```python
from build123d import *

# Parameters (mm, degrees)
BOSS_EXTRUDE1_DEPTH = 11.1125
BOSS_EXTRUDE2_DEPTH = 12.7
CUT_EXTRUDE2_DEPTH  = 8
CUT_EXTRUDE3_DEPTH  = 96.942967533
SKETCH5_W           = 25.144717139
SKETCH5_H           = 15.875
CUT_EXTRUDE4_DEPTH  = 3.175
CUT_EXTRUDE5_DEPTH  = 96.942967533
SKETCH6_R           = 2.54
CUT_EXTRUDE6_DEPTH  = 96.942967533
CUT_EXTRUDE7_START  = -3.175
CUT_EXTRUDE7_DEPTH  = 3.175
CHAMFER1_SIZE       = 3.175
FILLET1_R           = 0.635
FILLET3_R           = 1.016
SKETCH8_R           = 2.286
CUT_EXTRUDE8_DEPTH  = 93.295392221


with BuildPart() as part:
    # Sketch3 → Boss-Extrude1 (new, symmetric)
    with BuildSketch(Plane(origin=(0, 0, 0), x_dir=(1, 0, 0), z_dir=(0, 1, 0))):
        Polygon((-56.934473853, -15.948934871), (-65.016704362, -7.866704362), (-82.294717139, -25.144717139), (-74.93090712, -32.508527158), (-74.21248663, -33.226947648), align=None)
        Polygon((-65.016704362, -7.866704362), (-55.873813681, -17.009595043), (-52.371513794, -13.507295156), (-61.514404475, -4.364404475), align=None)
        Polygon((-52.371513794, -13.507295156), (-51.564218639, -12.7), (-17.311249955, -12.7), (0, -12.7), (0, 0), (-17.311249955, 0), (-57.15, 0), (-60.325, -3.175), (-61.514404475, -4.364404475), align=None)
        Polygon((0, 0), (0, -12.7), (17.311249955, -12.7), (51.564218639, -12.7), (52.371513794, -13.507295156), (61.514404475, -4.364404475), (60.325, -3.175), (57.15, 0), (17.311249955, 0), align=None)
        Polygon((61.514404475, -4.364404475), (65.016704362, -7.866704362), (55.873813681, -17.009595043), (52.371513794, -13.507295156), align=None)
        Polygon((65.016704362, -7.866704362), (56.934473853, -15.948934871), (74.21248663, -33.226947648), (74.93090712, -32.508527158), (82.294717139, -25.144717139), align=None)
    extrude(amount=BOSS_EXTRUDE1_DEPTH, both=True)

    # Sketch2 → Boss-Extrude2 (add)
    with BuildSketch(Plane.XY):
        with BuildLine():
            Line((-50.804788276, 11.1125), (50.804788276, 11.1125))
            Line((50.804788276, 11.1125), (8.344749207, 34.318436746))
            ThreePointArc((8.344749207, 34.318436746), (0, 36.45), (-8.344749207, 34.318436746))
            Line((-8.344749207, 34.318436746), (-50.804788276, 11.1125))
        make_face()
    extrude(amount=BOSS_EXTRUDE2_DEPTH)

    # Sketch2<3> → Cut-Extrude2 (cut)
    with BuildSketch(Plane.XY):
        with BuildLine():
            ThreePointArc((0, 30.1), (-11.05, 19.05), (0, 8))
            Line((0, 8), (0, 10))
            ThreePointArc((0, 10), (-9.05, 19.05), (0, 28.1))
            Line((0, 28.1), (0, 30.1))
        make_face()
        with BuildLine():
            Line((0, 10), (0, 8))
            ThreePointArc((0, 8), (7.813529932, 11.236470068), (11.05, 19.05))
            ThreePointArc((11.05, 19.05), (7.813529932, 26.863529932), (0, 30.1))
            Line((0, 30.1), (0, 28.1))
            ThreePointArc((0, 28.1), (6.39931637, 25.44931637), (9.05, 19.05))
            ThreePointArc((9.05, 19.05), (6.39931637, 12.65068363), (0, 10))
        make_face()
        with BuildLine():
            ThreePointArc((0, 28.1), (-9.05, 19.05), (0, 10))
            Line((0, 10), (0, 28.1))
        make_face()
        with BuildLine():
            Line((0, 28.1), (0, 10))
            ThreePointArc((0, 10), (6.39931637, 12.65068363), (9.05, 19.05))
            ThreePointArc((9.05, 19.05), (6.39931637, 25.44931637), (0, 28.1))
        make_face()
    extrude(amount=CUT_EXTRUDE2_DEPTH, mode=Mode.SUBTRACT)

    # Sketch2<5> → Cut-Extrude3 (cut, through all)
    with BuildSketch(Plane.XY):
        with BuildLine():
            ThreePointArc((0, 28.1), (-9.05, 19.05), (0, 10))
            Line((0, 10), (0, 28.1))
        make_face()
        with BuildLine():
            Line((0, 28.1), (0, 10))
            ThreePointArc((0, 10), (6.39931637, 12.65068363), (9.05, 19.05))
            ThreePointArc((9.05, 19.05), (6.39931637, 25.44931637), (0, 28.1))
        make_face()
    extrude(amount=CUT_EXTRUDE3_DEPTH, mode=Mode.SUBTRACT)

    # Sketch5 → Cut-Extrude4 (cut)
    # profile 1 of 5: a face of its own
    with BuildSketch(Plane(origin=(0, 0, 0), x_dir=(-1, 0, 0), z_dir=(0, 0, -1))):
        with Locations((-69.72235857, 3.175)):
            Rectangle(SKETCH5_W, SKETCH5_H)
    # profile 2 of 5: a face of its own
    with BuildSketch(Plane(origin=(0, 0, 0), x_dir=(-1, 0, 0), z_dir=(0, 0, -1))):
        with BuildLine():
            Line((-50.190202202, -4.7625), (-16.534774751, 13.631400187))
            ThreePointArc((-16.534774751, 13.631400187), (-16.178258512, 25.454994263), (-8.344749207, 34.318436746))
            Line((-8.344749207, 34.318436746), (-50.804788276, 11.1125))
            Line((-50.804788276, 11.1125), (-57.15, 11.1125))
            Line((-57.15, 11.1125), (-57.15, -4.7625))
            Line((-57.15, -4.7625), (-50.190202202, -4.7625))
        make_face()
    # profile 3 of 5: a face of its own
    with BuildSketch(Plane(origin=(0, 0, 0), x_dir=(-1, 0, 0), z_dir=(0, 0, -1))):
        with BuildLine():
            Line((50.804788276, 11.1125), (8.344749207, 34.318436746))
            ThreePointArc((8.344749207, 34.318436746), (14.965938597, 27.925848236), (17.4, 19.05))
            ThreePointArc((17.4, 19.05), (17.182332215, 16.306378367), (16.534774751, 13.631400187))
            Line((16.534774751, 13.631400187), (50.190202202, -4.7625))
            Line((50.190202202, -4.7625), (57.15, -4.7625))
            Line((57.15, -4.7625), (57.15, 11.1125))
            Line((57.15, 11.1125), (50.804788276, 11.1125))
        make_face()
    # profile 4 of 5: a face of its own
    with BuildSketch(Plane(origin=(0, 0, 0), x_dir=(-1, 0, 0), z_dir=(0, 0, -1))):
        with Locations((69.72235857, 3.175)):
            Rectangle(SKETCH5_W, SKETCH5_H)
    # profile 5 of 5: a face of its own
    with BuildSketch(Plane(origin=(0, 0, 0), x_dir=(-1, 0, 0), z_dir=(0, 0, -1))):
        with BuildLine():
            ThreePointArc((13.489420874, 8.059298271), (0, 1.65), (-13.489420874, 8.059298271))
            Line((-13.489420874, 8.059298271), (-41.5969936, -7.3025))
            Line((-41.5969936, -7.3025), (41.5969936, -7.3025))
            Line((41.5969936, -7.3025), (13.489420874, 8.059298271))
        make_face()
        with BuildLine():
            Line((31.653276027, -4.7625), (-31.653276027, -4.7625))
            Line((-31.653276027, -4.7625), (-14.022402602, 4.873405723))
            ThreePointArc((-14.022402602, 4.873405723), (0, -0.89), (14.022402602, 4.873405723))
            Line((14.022402602, 4.873405723), (31.653276027, -4.7625))
        make_face(mode=Mode.SUBTRACT)
    extrude(amount=-CUT_EXTRUDE4_DEPTH, mode=Mode.SUBTRACT)

    # Sketch5<3> → Cut-Extrude5 (cut, through all)
    with BuildSketch(Plane(origin=(0, 0, 0), x_dir=(-1, 0, 0), z_dir=(0, 0, -1))):
        with BuildLine():
            ThreePointArc((-14.022402602, 4.873405723), (0, -0.89), (14.022402602, 4.873405723))
            Line((14.022402602, 4.873405723), (31.653276027, -4.7625))
            Line((31.653276027, -4.7625), (-31.653276027, -4.7625))
            Line((-31.653276027, -4.7625), (-14.022402602, 4.873405723))
        make_face()
    extrude(amount=-CUT_EXTRUDE5_DEPTH, mode=Mode.SUBTRACT)

    # Sketch6 → Cut-Extrude6 (cut, through all)
    with BuildSketch(Plane(origin=(0, 0, 0), x_dir=(-1, 0, 0), z_dir=(0, 0, -1))):
        with Locations((-18.945146514, 8.695796817)):
            Circle(SKETCH6_R)
        with Locations((18.945146514, 8.695796817)):
            Circle(SKETCH6_R)
    extrude(amount=-CUT_EXTRUDE6_DEPTH, mode=Mode.SUBTRACT)

    # Sketch7 → Cut-Extrude7 (cut)
    # profile 1 of 3: a face of its own
    with BuildSketch(Plane.XY.offset(12.7).offset(CUT_EXTRUDE7_START)):
        with BuildLine():
            ThreePointArc((13.489420874, 8.059298271), (0, 1.65), (-13.489420874, 8.059298271))
            Line((-13.489420874, 8.059298271), (-41.5969936, -7.3025))
            Line((-41.5969936, -7.3025), (41.5969936, -7.3025))
            Line((41.5969936, -7.3025), (13.489420874, 8.059298271))
        make_face()
        with BuildLine():
            Line((-31.653276027, -4.7625), (-14.022402602, 4.873405723))
            ThreePointArc((-14.022402602, 4.873405723), (0, -0.89), (14.022402602, 4.873405723))
            Line((14.022402602, 4.873405723), (31.653276027, -4.7625))
            Line((31.653276027, -4.7625), (-31.653276027, -4.7625))
        make_face(mode=Mode.SUBTRACT)
    # profile 2 of 3: a face of its own
    with BuildSketch(Plane.XY.offset(12.7).offset(CUT_EXTRUDE7_START)):
        with BuildLine():
            Line((-51.564218639, -4.7625), (-50.190202202, -4.7625))
            Line((-50.190202202, -4.7625), (-16.534774751, 13.631400187))
            ThreePointArc((-16.534774751, 13.631400187), (-16.178258512, 25.454994263), (-8.344749207, 34.318436746))
            Line((-8.344749207, 34.318436746), (-50.804788276, 11.1125))
            Line((-50.804788276, 11.1125), (-51.564218639, 11.1125))
            Line((-51.564218639, 11.1125), (-51.564218639, -4.7625))
        make_face()
    # profile 3 of 3: a face of its own
    with BuildSketch(Plane.XY.offset(12.7).offset(CUT_EXTRUDE7_START)):
        with BuildLine():
            Line((50.804788276, 11.1125), (8.344749207, 34.318436746))
            ThreePointArc((8.344749207, 34.318436746), (14.965938597, 27.925848236), (17.4, 19.05))
            ThreePointArc((17.4, 19.05), (17.182332215, 16.306378367), (16.534774751, 13.631400187))
            Line((16.534774751, 13.631400187), (50.190202202, -4.7625))
            Line((50.190202202, -4.7625), (51.564218639, -4.7625))
            Line((51.564218639, -4.7625), (51.564218639, 11.1125))
            Line((51.564218639, 11.1125), (50.804788276, 11.1125))
        make_face()
    extrude(amount=CUT_EXTRUDE7_DEPTH, mode=Mode.SUBTRACT)

    # Chamfer1
    chamfer1_edges = [part.edges().sort_by_distance(p)[0] for p in [
        (51.564218639, 3.175, 9.525),
        (-51.564218639, 3.175, 9.525),
    ]]
    chamfer(chamfer1_edges, length=CHAMFER1_SIZE - 0.0001)  # a hair under: the kernel refuses the full size

    # Fillet1
    fillet1_edges = [part.edges().sort_by_distance(p)[0] for p in [
        (13.489420874, 8.059298271, 1.5875),
        (-13.489420874, 8.059298271, 1.5875),
        (-41.5969936, -7.3025, 1.5875),
        (41.5969936, -7.3025, 1.5875),
        (14.022402602, 4.873405723, 6.35),
        (31.653276027, -4.7625, 6.35),
        (-31.653276027, -4.7625, 6.35),
        (-14.022402602, 4.873405723, 6.35),
        (-13.489420874, 8.059298271, 11.1125),
        (13.489420874, 8.059298271, 11.1125),
        (41.5969936, -7.3025, 11.1125),
        (-41.5969936, -7.3025, 11.1125),
    ]]
    fillet(fillet1_edges, radius=FILLET1_R)

    # Fillet3
    fillet3_edges = [part.edges().sort_by_distance(p)[0] for p in [
        (65.573480242, -11.1125, 24.587941259),
        (-65.573480242, -11.1125, 24.587941259),
        (65.573480242, 11.1125, 24.587941259),
        (-65.573480242, 11.1125, 24.587941259),
    ]]
    fillet(fillet3_edges, radius=FILLET3_R)

    # Sketch8 → Cut-Extrude8 (cut, through all)
    with BuildSketch(Plane(origin=(0, 11.1125, 0), x_dir=(1, 0, 0), z_dir=(0, 1, 0))):
        with Locations(Location((74.625578412, -25.198598676, 0), (0, 0, 270))):
            Circle(SKETCH8_R)
        with Locations(Location((-74.625578412, -25.198598676, 0), (0, 0, 270))):
            Circle(SKETCH8_R)
        with Locations(Location((65.645322291, -16.218342555, 0), (0, 0, 270))):
            Circle(SKETCH8_R)
        with Locations(Location((-65.645322291, -16.218342555, 0), (0, 0, 90))):
            Circle(SKETCH8_R)
    extrude(amount=-CUT_EXTRUDE8_DEPTH, mode=Mode.SUBTRACT)


solid = part.part
```
Design review of the part built by this model. Coordinates are the model's own, in mm. A direction names the side the tool comes from. Round coordinates to 2 decimals unless told otherwise and drop trailing zeros. Write each loop counter-clockwise with the first axis right and the second up, starting at its lowest first coordinate (ties: lowest second). Pieces come first, ordered by that corner, then holes.
Item 1: We need section C-C on z = 6. State how many separate pieces and enclosed holes the cut face has, and give its area (3 significant figures).
Item 2: Clearance check with flat-ended pins moving along their axes: pin 1 Ø4 at (x, y) = (39, 13.5) entering from -Z (3 decimals); pin 2 Ø24 at (x, y) = (-2, 21) entering from +Z; pin 3 Ø1.9 at (x, z) = (-7, 6) entering from +Y. State where each tip first meets the part, or that it passes through.
Item 3: We need section A-A on y = 22. Write out the cut boundary in (x, z) (3 decimals), and give its area (3 significant figures).
Item 4: We need section B-B on x = -42.5. Write out the cut boundary in (y, z) (1 decimal).
Item 5: For probe 1 along Z at (x, y) = (-37.5, 17) (3 decimals); probe 2 along Z at (x, y) = (10, 28); probe 3 along X at (y, z) = (9, 15), list the stretches that pass through material, from the lowest coordinate up.
Item 6: For faces 1 (the flat face through (-65.694, 0.141, 24.709)), 2 (the cylindrical face through (65.91, 10.823, 24.493)), 3 (the flat face through (-21.847, 0.597, 6.306)), list the 3-axis set-ups (+Z, -Z, +X, -X, +Y, -Y) from which the entire face can be reached by the end or side of a thin tool; tool diameter is ignored.
Item 7: The part is to be moulded in two halves that separate along Y. For faces 4 (the flat face through (-26.86, 0.75, 1.57)), 5 (the flat face through (-69.55, 0.16, 12.4)), 6 (the flat face through (-63, 11.112, 18)), 7 (the flat face through (22.06, 0.48, 6.31)), say which applies: +Y half, -Y half, draft (parallel to the pull), parting line (faces both ways), or undercut.
Returned:
1. separate pieces: 1
1. enclosed holes: 4
1. area: 3,450 mm2
2. pin 1: stops at z = 3.175
2. pin 2: stops at z = 12.7
2. pin 3: stops at y = 35.36
3. outline: (-30.884, 3.175) - (-17.148, 3.175) - (-17.148, 0) - (-10.649, 0) - (-10.649, 8) - (-8.556, 8) - (-8.556, 12.7) - (-17.148, 12.7) - (-17.148, 9.525) - (-30.884, 9.525) - close; (8.556, 8) - (10.649, 8) - (10.649, 0) - (17.148, 0) - (17.148, 3.175) - (30.884, 3.175) - (30.884, 9.525) - (17.148, 9.525) - (17.148, 12.7) - (8.556, 12.7) - close
3. area: 359 mm2
4. outline: (-11.1, 0) - (-0.6, 0) - (-0.6, 3.2) - (15.7, 3.2) - (15.7, 9.5) - (-0.6, 9.5) - (-0.6, 12.7) - (-11.1, 12.7) - close
5. probe 1: z = 3.175 to 9.525
5. probe 2: z = 0 to 12.7
5. probe 3: x = -72.15 to -67.58, -63.71 to -53.86, 53.86 to 63.71, 67.58 to 72.15
6. face 1: +Z, +Y, -Y
6. face 2: +Z, +Y
6. face 3: +Z, -Z
7. face 4: undercut
7. face 5: draft
7. face 6: +Y half
7. face 7: undercut
